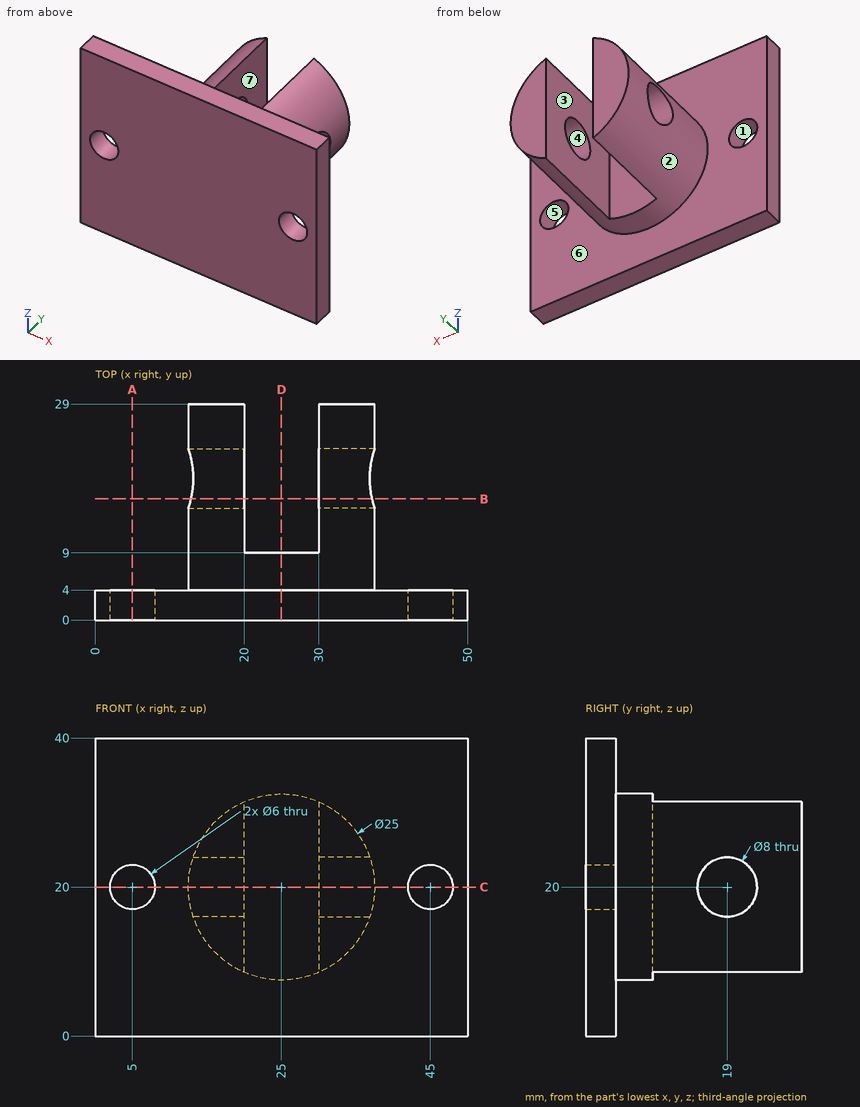
The drawing under review shows one solid part. Ordinate dimensions are in mm from its lowest x, y, z. A direction names the side the tool comes from. Coordinates: 2 decimals unless noted, no trailing zeros. Write each loop counter-clockwise with the first axis right and the second up, starting at its lowest first coordinate (ties: lowest second). Pieces come first, ordered by that corner, then holes. Notation, with made-up numbers: (53, 70) -> (91, 70) arc R26 ccw to (91, 88) -> close; hole circle Ø9 at (-10.5, 78). An arc over 180 degrees is marked (long way). One line per item, written item: value. Start each with the question number.
Q1. The part is to be moulded in two halves that separate along Z. For the marked faces 1, 2, 3 and 4, say which applies: +Z half, -Z half, draft (parallel to the pull), parting line (faces both ways), or undercut.
Q2. To check wall thickness, follow probe 1 along X at (y, z) = (1.85, 20); probe 2 along Y at (x, z) = (14, 20); probe 3 along Y at (x, z) = (27.5, 26). State the ranges of each line that lie inside material, in increasing order.
Q3. Add section B-B, the plane y = 16.25. Give the boundary of the cut face in (x, z), then the cut area to 3 significant figures.
Q4. Add section C-C, the plane z = 20. Give the boundary of the cut face in (x, y), then the cut area to 3 significant figures.
Q5. Add section D-D, the plane x = 25. Give the boundary of the cut face in (y, z), then the cut area to 3 significant figures.
Q6. Add section A-A, the plane x = 5. Give the boundary of the cut face in (y, z).
Q7. For the marked faces 5, 6 and 7, list the 3-axis set-ups (+Z, -Z, +X, -X, +Y, -Y) from which the entire face can be reached by the end or side of a thin tool; tool diameter is ignored.
Q8. Clearance check with flat-ended pins moving along their axes: P1, Ø5, axis at x = 5, z = 20, coming from the +Y side; P2, Ø6, axis at y = 18, z = 23.5, coming from the +X side; P3, Ø4, axis at x = 20.5, y = 19.5, coming from the -Z side; P4, Ø1, axis at y = 21, z = 13, coming from the -X side. State where each tip first meets the part, or that it passes through.
Response:
1. face 1: undercut
1. face 2: parting line
1. face 3: draft
1. face 4: undercut
2. probe 1: 0 to 2, 8 to 42, 48 to 50
2. probe 2: 0 to 15, 23 to 29
2. probe 3: 0 to 9
3. outline: (12.84, 17.1) arc R12.5 ccw to (20, 8.54) -> (20, 17.1) -> close; (12.84, 22.9) -> (20, 22.9) -> (20, 31.46) arc R12.5 ccw to start; (30, 8.54) arc R12.5 ccw to (37.16, 17.1) -> (30, 17.1) -> close; (30, 22.9) -> (37.16, 22.9) arc R12.5 ccw to (30, 31.46) -> close
3. area: 162 mm²
4. outline: (0, 0) -> (2, 0) -> (2, 4) -> (0, 4) -> close; (8, 0) -> (42, 0) -> (42, 4) -> (37.5, 4) -> (37.5, 15) -> (30, 15) -> (30, 9) -> (20, 9) -> (20, 15) -> (12.5, 15) -> (12.5, 4) -> (8, 4) -> close; (12.5, 23) -> (20, 23) -> (20, 29) -> (12.5, 29) -> close; (30, 23) -> (37.5, 23) -> (37.5, 29) -> (30, 29) -> close; (48, 0) -> (50, 0) -> (50, 4) -> (48, 4) -> close
4. area: 457 mm²
5. outline: (0, 0) -> (4, 0) -> (4, 7.5) -> (9, 7.5) -> (9, 32.5) -> (4, 32.5) -> (4, 40) -> (0, 40) -> close
5. area: 285 mm²
6. outline: (0, 0) -> (4, 0) -> (4, 17) -> (0, 17) -> close; (0, 23) -> (4, 23) -> (4, 40) -> (0, 40) -> close
7. face 5: +Y, -Y
7. face 6: +Y
7. face 7: +Z, -Z, +Y
8. P1: through
8. P2: x = 37.36
8. P3: z = 8.54
8. P4: x = 14.32
